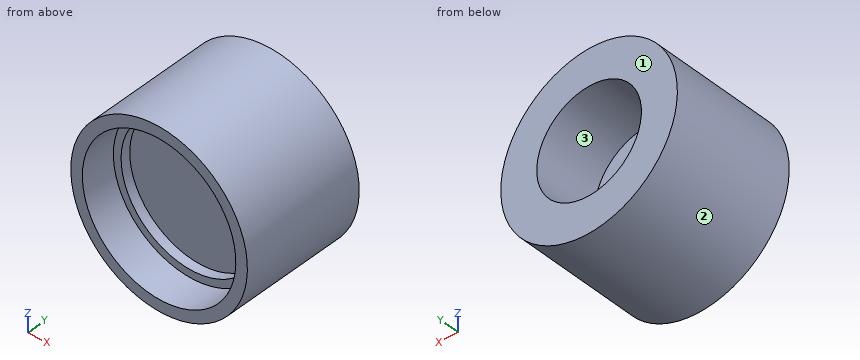
from build123d import *

# Parameters (mm, degrees)
SKETCH1_R           = 27.5
SKETCH1_R_2         = 23.9
BOSS_EXTRUDE1_DEPTH = 10.75
SKETCH2_R           = 27.5
SKETCH2_R_2         = 21.5
BOSS_EXTRUDE2_DEPTH = 3
SKETCH3_R           = 27.5
BOSS_EXTRUDE3_DEPTH = 5
SKETCH4_R           = 27.5
SKETCH4_R_2         = 16.3
BOSS_EXTRUDE4_DEPTH = 20


with BuildPart() as part:
    # Sketch1 → Boss-Extrude1 (new body)
    with BuildSketch(Plane(origin=(0, 0, 0), x_dir=(1, 0, 0), z_dir=(0, 1, 0))):
        with Locations(Location((0, 0, 0), (0, 0, 270))):
            Circle(SKETCH1_R)
        with Locations(Location((0, 0, 0), (0, 0, 270))):
            Circle(SKETCH1_R_2, mode=Mode.SUBTRACT)
    extrude(amount=BOSS_EXTRUDE1_DEPTH)

    # Sketch2 → Boss-Extrude2 (add)
    with BuildSketch(Plane(origin=(0, 10.75, 0), x_dir=(1, 0, 0), z_dir=(0, 1, 0))):
        with Locations(Location((0, 0, 0), (0, 0, 270))):
            Circle(SKETCH2_R)
        with Locations(Location((0, 0, 0), (0, 0, 270))):
            Circle(SKETCH2_R_2, mode=Mode.SUBTRACT)
    extrude(amount=BOSS_EXTRUDE2_DEPTH)

    # Sketch3 → Boss-Extrude3 (add)
    with BuildSketch(Plane(origin=(0, 13.75, 0), x_dir=(1, 0, 0), z_dir=(0, 1, 0))):
        with Locations(Location((0, 0, 0), (0, 0, 270))):
            Circle(SKETCH3_R)
    extrude(amount=BOSS_EXTRUDE3_DEPTH)

    # Sketch4 → Boss-Extrude4 (add)
    with BuildSketch(Plane(origin=(0, 18.75, 0), x_dir=(1, 0, 0), z_dir=(0, 1, 0))):
        with Locations(Location((0, 0, 0), (0, 0, 270))):
            Circle(SKETCH4_R)
        with Locations(Location((0, 0, 0), (0, 0, 270))):
            Circle(SKETCH4_R_2, mode=Mode.SUBTRACT)
    extrude(amount=BOSS_EXTRUDE4_DEPTH)


solid = part.part
Model file for the job. Use its own axes, mm. Face numbers are marked on the shaded views. Give positions to 0.01 mm unless a question says otherwise; leave off trailing zeros. Loops run counter-clockwise (first coordinate to the right, second up) from the corner with the lowest first, then second, coordinate; pieces in that order, holes last. Notation, with made-up numbers: (1, -17) - (17, -17) arc R34 cw to (17, 17) - close; hole circle Ø10 at (-17.5, 82.25). An arc over 180 degrees is marked (long way). Use one line per item in the form item = value.
(1) Cut at D-D (y = 15). Give the cut face in (x, z).
Determined:
outline = circle Ø55 at (0, 0)
(2) Pull direction Z, two halves, no side cores. Call the marked faces 1, 2 and 3: pulls with the +Z half, pulls with the -Z half, needs draft (parallel to the pull), parting line crosses it, or undercut.
Determined:
face_1 = needs draft
face_2 = parting line crosses it
face_3 = undercut
(3) Cut at B-B (z = 0). Give the cut face in (x, y), then the cut area to 3 significant figures.
Determined:
outline = (-27.5, 0) - (-23.9, 0) - (-23.9, 10.75) - (-21.5, 10.75) - (-21.5, 13.75) - (21.5, 13.75) - (21.5, 10.75) - (23.9, 10.75) - (23.9, 0) - (27.5, 0) - (27.5, 38.75) - (16.3, 38.75) - (16.3, 18.75) - (-16.3, 18.75) - (-16.3, 38.75) - (-27.5, 38.75) - close
area = 836 mm^2
(4) Cut at C-C (y = 32.5). Give the cut face in (x, z), then the cut area to 3 significant figures.
Determined:
outline = circle Ø55 at (0, 0); hole circle Ø32.6 at (0, 0)
area = 1,540 mm^2
(5) Cut at A-A (x = 0). Give the cut face in (y, z), then the cut area to 3 significant figures.
Determined:
outline = (0, -27.5) - (38.75, -27.5) - (38.75, -16.3) - (18.75, -16.3) - (18.75, 16.3) - (38.75, 16.3) - (38.75, 27.5) - (0, 27.5) - (0, 23.9) - (10.75, 23.9) - (10.75, 21.5) - (13.75, 21.5) - (13.75, -21.5) - (10.75, -21.5) - (10.75, -23.9) - (0, -23.9) - close
area = 836 mm^2
(6) Drop flat-ended pins along their axis: P1, Ø21.5, axis at x = -1.5, z = 9, coming from the -Y side; P2, Ø1.5, axis at x = 12, y = 4, coming from the -Z side; P3, Ø10, axis at x = 8, z = 1.5, coming from the +Y side. Give the stop position or say it passes through.
Determined:
P1 = 13.75
P2 = -25.09
P3 = 18.75
(7) Drill centre lines: L1, parallel to X at y = 22, z = -0.5; L2, parallel to X at y = 5.25, z = 0; L3, parallel to Y at x = -15.5, z = 1.5. Where is each one in solid material? Low to high.
Determined:
L1 = -27.5 to -16.29, 16.29 to 27.5
L2 = -27.5 to -23.9, 23.9 to 27.5
L3 = 13.75 to 18.75
